Here's how the part is built. I have some questions about the finished solid (model axes, mm). Face numbers are marked on the shaded views. A direction names the side the tool comes from. Give positions to 0.01 mm unless a question says otherwise; leave off trailing zeros. Order: outer loops, then holes, each group sorted by start corner. A loop starts at its lowest first (then second) coordinate and runs counter-clockwise, first axis right, second up. Notation, with made-up numbers: (72, 73.25) -> (126, 73.25) arc R13 ccw to (126, 85.25) -> close; hole circle Ø2 at (65.25, -9.5). An arc over 180 degrees is marked (long way). Write each question's results on one line, items separated by ' | '. Start each with the question number.
Q1. Thinking about a two-plate mould opening in Z: for the marked faces 3, 4, 5 and 6, which applies, pulls with the +Z half, pulls with the -Z half, needs draft (parallel to the pull), parting line crosses it, or undercut?
Q2. Imagine slicing it at D-D, the plane x = 11. Please give me the cut outline in (y, z), then the cut area to 3 significant figures.
Q3. Imagine slicing it at B-B, the plane z = -13. Please give me the cut outline in (x, y) (1 decimal).
Q4. Imagine slicing it at A-A, the plane x = 18. Please give me the cut outline in (y, z).
Q5. For the marked faces 1 and 2, which set-ups out of +Z, -Z, +X, -X, +Y, -Y let a thin tool reach every point of the face, with its end or its side?
Q6. I'm going to push flat-ended pins straight in: pin 1 (6 mm diameter, centred on x = -6, z = 7.5, fed in from +Y); pin 2 (5 mm diameter, centred on x = 16, z = 11, fed in from +Y). Where does each tip first touch, or does it pass through?
Q7. I need wall thicknesses on line 1 along X through (y, z) = (1, -13.5); line 2 along Z through (x, y) = (19, 0.5); line 3 along X through (y, z) = (1, -15.5). Which ranges of each line are inside material? Lowest first, please. Write a range as [from, to].
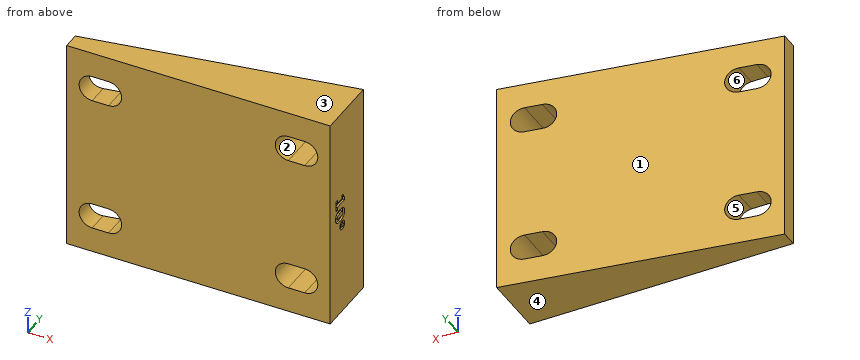
Autodesk Inventor part; units mm, degrees
ref_plane "YZ Plane" through (0, 0, 0) normal (1, 0, 0) x (0, 1, 0)
ref_plane "XZ Plane" through (0, 0, 0) normal (0, 1, 0) x (-1, 0, 0)
ref_plane "XY Plane" through (0, 0, 0) normal (0, 0, 1) x (1, 0, 0)
sketch "Sketch1" plane through (0, 0, 0) normal (0, 1, 0) x (-1, 0, 0)
  line L0 (25.527, 20.828) -> (-25.527, 20.828)
  line L1 (-25.527, 20.828) -> (-25.527, -20.828)
  line L2 (-25.527, -20.828) -> (25.527, -20.828)
  line L3 (25.527, -20.828) -> (25.527, 20.828)
  circle A0 centre (18.9992, 13.3858) radius 1.9837
  circle A1 centre (18.9992, -13.3858) radius 1.9837
  circle A2 centre (-18.9992, -13.3858) radius 1.9837
  circle A3 centre (-18.9992, 13.3858) radius 1.9837
  circle A4 centre (18.9992, 13.3858) radius 3.048 construction
  point P0 (0, 0)
  point P1 (25.527, 0)
  point P2 (0, -20.828)
  dimension "d0" = 3.9675
  dimension "d1" = 41.656
  dimension "d2" = 51.054
  dimension "d3" = 6.096
  dimension "d4" = 7.4422
  dimension "d5" = 6.5278
  dimension "d6" = 7.4422
  dimension "d7" = 6.5278
sketch "Sketch10" plane through (0, 0, 0) normal (0, 0, 1) x (1, 0, 0)
  line L0 (-25.527, 0) -> (25.527, 0)
  line L1 (25.527, 0) -> (25.527, 12.1772)
  line L2 (-25.527, 0) -> (-25.527, 3.175)
  line L3 (-25.527, 3.175) -> (25.527, 12.1772)
  point P0 (0, 0)
  dimension "d61" = 10
  dimension "d62" = 3.175
extrude "Extrusion8" add sketch "Sketch10" along normal mid plane 41.656
sketch "Sketch11" plane through (-25.527, 0, 20.828) normal (0, -1, 0) x (1, 0, 0)
  line L0 (46.1137, -7.4422) -> (42.9387, -7.4422) construction
  line L1 (46.1137, -4.9149) -> (42.9387, -4.9149)
  line L2 (42.9387, -9.9695) -> (46.1137, -9.9695)
  arc A0 (46.1137, -9.9695) -> (46.1137, -4.9149) centre (46.1137, -7.4422) ccw
  arc A1 (42.9387, -4.9149) -> (42.9387, -9.9695) centre (42.9387, -7.4422) ccw
  line L3 (46.1137, -34.2138) -> (42.9387, -34.2138) construction
  line L4 (51.054, -41.656) -> (51.054, 0)
  line L5 (46.1137, -36.7411) -> (42.9387, -36.7411)
  line L6 (42.9387, -31.6865) -> (46.1137, -31.6865)
  arc A2 (46.1137, -36.7411) -> (46.1137, -31.6865) centre (46.1137, -34.2138) ccw
  arc A3 (42.9387, -31.6865) -> (42.9387, -36.7411) centre (42.9387, -34.2138) ccw
  line L7 (8.1153, -34.2138) -> (4.9403, -34.2138) construction
  line L8 (8.1153, -36.7411) -> (4.9403, -36.7411)
  line L9 (4.9403, -31.6865) -> (8.1153, -31.6865)
  arc A4 (8.1153, -36.7411) -> (8.1153, -31.6865) centre (8.1153, -34.2138) ccw
  arc A5 (4.9403, -31.6865) -> (4.9403, -36.7411) centre (4.9403, -34.2138) ccw
  line L10 (8.1153, -7.4422) -> (4.9403, -7.4422) construction
  line L11 (8.1153, -9.9695) -> (4.9403, -9.9695)
  line L12 (4.9403, -4.9149) -> (8.1153, -4.9149)
  arc A6 (8.1153, -9.9695) -> (8.1153, -4.9149) centre (8.1153, -7.4422) ccw
  arc A7 (4.9403, -4.9149) -> (4.9403, -9.9695) centre (4.9403, -7.4422) ccw
  point P0 (25.527, -20.828)
  point P1 (44.5262, -7.4422)
  point P2 (44.5262, -34.2138)
  point P3 (6.5278, -34.2138)
  point P4 (6.5278, -7.4422)
  point P5 (44.5262, -7.4422)
  point P6 (44.5262, -34.2138)
  point P7 (6.5278, -34.2138)
  point P8 (6.5278, -7.4422)
  point P9 (44.5262, -9.9695)
  point P10 (6.5278, -36.7411)
  dimension "d65" = 3.175
  dimension "d66" = 2.5273
extrude "Extrusion9" cut sketch "Sketch11" against normal blind 41.656
sketch "Sketch13" plane through (25.527, 0, 20.828) normal (1, 0, 0) x (0, 0, -1)
  line L0 (41.656, 12.1772) -> (0, 12.1772)
  line L1 (0, 0) -> (0, 12.1772)
  line L2 (41.656, 0) -> (0, 0)
  line L3 (41.656, 12.1772) -> (41.656, 0)
  line L4 (25.4999, 2.032) -> (16.1561, 2.032)
  line L5 (19.4258, 2.032) -> (17.3288, 2.032)
  line L6 (17.3288, 2.032) -> (17.3288, 2.5852)
  line L7 (17.3288, 2.5852) -> (17.9978, 2.5852)
  line L8 (17.9978, 2.5852) -> (17.9978, 4.2653)
  line L9 (17.9978, 4.2653) -> (17.3288, 4.2653)
  line L10 (17.3288, 4.2653) -> (17.3288, 4.7825)
  spline S0 degree 2 poles (17.3288, 4.7825) (17.4755, 4.7825) (17.7662, 4.8211) (17.8537, 4.8622) knots 0 0 0 1 2 2 2
  spline S1 degree 2 poles (17.8537, 4.8622) (17.954, 4.9137) (18.0672, 5.0861) (18.0775, 5.2147) knots 0 0 0 1 2 2 2
  line L11 (18.0775, 5.2147) -> (18.7722, 5.2147)
  line L12 (18.7722, 5.2147) -> (18.7722, 2.5852)
  line L13 (18.7722, 2.5852) -> (19.4258, 2.5852)
  line L14 (19.4258, 2.5852) -> (19.4258, 2.032)
  spline S2 degree 2 poles (22.3074, 3.6195) (22.3074, 3.2078) (22.1762, 2.5903) (22.0296, 2.3819) knots 0 0 0 1 2 2 2
  spline S3 degree 2 poles (22.0296, 2.3819) (21.8855, 2.1761) (21.4198, 1.9651) (21.0853, 1.9651) knots 0 0 0 1 2 2 2
  spline S4 degree 2 poles (21.0853, 1.9651) (20.7482, 1.9651) (20.2851, 2.1761) (20.1385, 2.3871) knots 0 0 0 1 2 2 2
  spline S5 degree 2 poles (20.1385, 2.3871) (19.9918, 2.5955) (19.8606, 3.2078) (19.8606, 3.6195) knots 0 0 0 1 2 2 2
  spline S6 degree 2 poles (19.8606, 3.6195) (19.8606, 4.0415) (19.9918, 4.6384) (20.141, 4.8545) knots 0 0 0 1 2 2 2
  spline S7 degree 2 poles (20.141, 4.8545) (20.2903, 5.0655) (20.7611, 5.2713) (21.0853, 5.2713) knots 0 0 0 1 2 2 2
  spline S8 degree 2 poles (21.0853, 5.2713) (21.4275, 5.2713) (21.8855, 5.0552) (22.0321, 4.8416) knots 0 0 0 1 2 2 2
  spline S9 degree 2 poles (22.0321, 4.8416) (22.1762, 4.6332) (22.3074, 4.0183) (22.3074, 3.6195) knots 0 0 0 1 2 2 2
  spline S10 degree 2 poles (21.5073, 3.6195) (21.5073, 4.2087) (21.3143, 4.6847) (21.0853, 4.6847) knots 0 0 0 1 2 2 2
  spline S11 degree 2 poles (21.0853, 4.6847) (20.8563, 4.6847) (20.6608, 4.2087) (20.6608, 3.6169) knots 0 0 0 1 2 2 2
  spline S12 degree 2 poles (20.6608, 3.6169) (20.6608, 3.0354) (20.8563, 2.5517) (21.0853, 2.5517) knots 0 0 0 1 2 2 2
  spline S13 degree 2 poles (21.0853, 2.5517) (21.3117, 2.5517) (21.5073, 3.0354) (21.5073, 3.6195) knots 0 0 0 1 2 2 2
  spline S14 degree 2 poles (24.4738, 4.4145) (24.4738, 4.0518) (23.9696, 3.5552) (23.6093, 3.5552) knots 0 0 0 1 2 2 2
  spline S15 degree 2 poles (23.6093, 3.5552) (23.2466, 3.5552) (22.7423, 4.0518) (22.7423, 4.4145) knots 0 0 0 1 2 2 2
  spline S16 degree 2 poles (22.7423, 4.4145) (22.7423, 4.7773) (23.2466, 5.2739) (23.6093, 5.2739) knots 0 0 0 1 2 2 2
  spline S17 degree 2 poles (23.6093, 5.2739) (23.9721, 5.2739) (24.4738, 4.7773) (24.4738, 4.4145) knots 0 0 0 1 2 2 2
  spline S18 degree 2 poles (24.0081, 4.4145) (24.0081, 4.5818) (23.7792, 4.8211) (23.6093, 4.8211) knots 0 0 0 1 2 2 2
  spline S19 degree 2 poles (23.6093, 4.8211) (23.4395, 4.8211) (23.208, 4.5844) (23.208, 4.4145) knots 0 0 0 1 2 2 2
  spline S20 degree 2 poles (23.208, 4.4145) (23.208, 4.2396) (23.4421, 4.008) (23.6093, 4.008) knots 0 0 0 1 2 2 2
  spline S21 degree 2 poles (23.6093, 4.008) (23.7792, 4.008) (24.0081, 4.2447) (24.0081, 4.4145) knots 0 0 0 1 2 2 2
  point P0 (20.828, 0)
  point P1 (20.828, 0)
  point P2 (20.828, 2.032)
  dimension "d69" = 2.032
extrude "Extrusion10" cut sketch "Sketch13" against normal blind 0.381 contours S4 S5 S6 S7 S8 S9 S2 S3 L4 | L4 S3 S4 | L4 L6 L7 L8 L9 L10 S0 S1 L11 L12 L13 L14 | S14 S15 S16 S17
equation "\"d6\" = d4"
equation "\"d7\" = d5"
equation "\"d23\" = d22"
equation "\"d25\" = 0.5 * d24"
properties part number "shim 10 Deg"
Geometry check:
1) face 3: pulls with the +Z half | face 4: pulls with the -Z half | face 5: undercut | face 6: undercut
2) outline: (0, -20.83) -> (9.62, -20.83) -> (9.62, 20.83) -> (0, 20.83) -> close | area: 401 mm²
3) outline: (-25.5, 0) -> (-23.1, 0) -> (-23.1, 3.6) -> (-25.5, 3.2) -> close; (-14.9, 0) -> (14.9, 0) -> (14.9, 10.3) -> (-14.9, 5) -> close; (23.1, 0) -> (25.5, 0) -> (25.5, 12.2) -> (23.1, 11.7) -> close
4) outline: (0, -20.83) -> (10.85, -20.83) -> (10.85, -15.91) -> (0, -15.91) -> close; (0, -10.86) -> (10.85, -10.86) -> (10.85, 10.86) -> (0, 10.86) -> close; (0, 15.91) -> (10.85, 15.91) -> (10.85, 20.83) -> (0, 20.83) -> close
5) face 1: +Z, -Z, -X, +Y | face 2: +Y, -Y
6) pin 1: y = 7.15 | pin 2: y = 10.94
7) line 1: [-25.53, -23.11], [-14.89, 14.89], [23.11, 25.53] | line 2: [-20.83, -15.91], [-10.86, 10.86], [15.91, 20.83] | line 3: [-25.53, -21.97], [-16.03, 16.03], [21.97, 25.53]
